The listing builds one solid part. Answer for the finished solid, in the listing's coordinates (mm). Give positions to 0.01 mm unless a question says otherwise; leave off trailing zeros. Write each loop counter-clockwise with the first axis right and the second up, starting at its lowest first coordinate (ties: lowest second). Pieces come first, ordered by that corner, then holes. Notation, with made-up numbers: (51, -28.75) -> (73, -28.75) arc R20 ccw to (73, -11.75) -> close; hole circle Ø1 at (-31, 23). An arc over 180 degrees is marked (long way). One line per question, with ' | ' between items.
from build123d import *

# Parameters (mm, degrees)
SKETCH_1_R          = 1.75
SKETCH_1_R_2        = 1.5
EXTRUDE_1_DEPTH     = 2
SKETCH_2_W          = 27.7
SKETCH_2_H          = 5
CUT_EXTRUDE_1_DEPTH = 10
SKETCH_3_R          = 1.5
CUT_EXTRUDE_2_DEPTH = 10
SKETCH_4_W          = 70
SKETCH_4_H          = 3
EXTRUDE_2_DEPTH     = 2
FILLET_1_R          = 1


with BuildPart() as part:
    # 草图1 → 凸台-拉伸1 (new body)
    with BuildSketch(Plane.XY):
        with BuildLine():
            Line((-35, -27.810744327), (-35, -46.920144927))
            Line((-35, -46.920144927), (35, -46.920144927))
            Line((35, -46.920144927), (35, -27.810744327))
            ThreePointArc((35, -27.810744327), (16.334866743, -2.254950607), (30.958156738, 25.81006644))
            Line((30.958156738, 25.81006644), (35, 32.810744327))
            Line((35, 32.810744327), (35, 46.920144927))
            Line((35, 46.920144927), (16.8, 46.920144927))
            Line((16.8, 46.920144927), (16.8, 51.920144927))
            Line((16.8, 51.920144927), (-10.9, 51.920144927))
            Line((-10.9, 51.920144927), (-10.9, 46.920144927))
            Line((-10.9, 46.920144927), (-35, 46.920144927))
            Line((-35, 46.920144927), (-35, 32.810744327))
            Line((-35, 32.810744327), (-27, 28.191942173))
            Line((-27, 28.191942173), (-27, 23.009508904))
            ThreePointArc((-27, 23.009508904), (-16.614935725, -4.665079356), (-35, -27.810744327))
        make_face()
        with Locations((-16.1979618, -30.0520382)):
            Circle(SKETCH_1_R, mode=Mode.SUBTRACT)
        with Locations((-3.75, 0)):
            Circle(SKETCH_1_R, mode=Mode.SUBTRACT)
        with Locations((16.1979618, -30.0520382)):
            Circle(SKETCH_1_R, mode=Mode.SUBTRACT)
        with Locations((3.75, 0)):
            Circle(SKETCH_1_R, mode=Mode.SUBTRACT)
        with Locations((-16.1979618, 30.0520382)):
            Circle(SKETCH_1_R, mode=Mode.SUBTRACT)
        with Locations((-3.05, 40)):
            Circle(SKETCH_1_R_2, mode=Mode.SUBTRACT)
        with Locations((16.1979618, 30.0520382)):
            Circle(SKETCH_1_R, mode=Mode.SUBTRACT)
        with Locations((11.95, 40)):
            Circle(SKETCH_1_R_2, mode=Mode.SUBTRACT)
    extrude(amount=EXTRUDE_1_DEPTH)

    # 草图2 → 切除-拉伸1 (cut)
    with BuildSketch(Plane(origin=(0, 0, 0), x_dir=(-1, 0, 0), z_dir=(0, 0, -1))):
        with Locations((-2.95, 49.420144927)):
            Rectangle(SKETCH_2_W, SKETCH_2_H)
    extrude(amount=-CUT_EXTRUDE_1_DEPTH, mode=Mode.SUBTRACT)

    # 草图3 → 切除-拉伸2 (cut)
    with BuildSketch(Plane(origin=(0, 0, 0), x_dir=(-1, 0, 0), z_dir=(0, 0, -1))):
        with Locations((-15, 20)):
            Circle(SKETCH_3_R)
        with Locations((15, 20)):
            Circle(SKETCH_3_R)
        with Locations((15, -20)):
            Circle(SKETCH_3_R)
        with Locations((-15, -20)):
            Circle(SKETCH_3_R)
    extrude(amount=-CUT_EXTRUDE_2_DEPTH, mode=Mode.SUBTRACT)

    # 草图4 → 凸台-拉伸2 (add)
    with BuildSketch(Plane(origin=(0, 0, 0), x_dir=(-1, 0, 0), z_dir=(0, 0, -1))):
        with Locations((0, -48.420144927)):
            Rectangle(SKETCH_4_W, SKETCH_4_H)
    extrude(amount=-EXTRUDE_2_DEPTH)

    # 圆角1
    fillet_1_edges = [part.edges().sort_by_distance(p)[0] for p in [
        (35, -49.920144927, 1),
        (-35, -49.920144927, 1),
        (35, -27.810744327, 1),
        (-35, -27.810744327, 1),
        (-27, 23.009508904, 1),
        (-35, 32.810744327, 1),
        (-35, 46.920144927, 1),
        (35, 46.920144927, 1),
    ]]
    fillet(fillet_1_edges, radius=FILLET_1_R)


solid = part.part
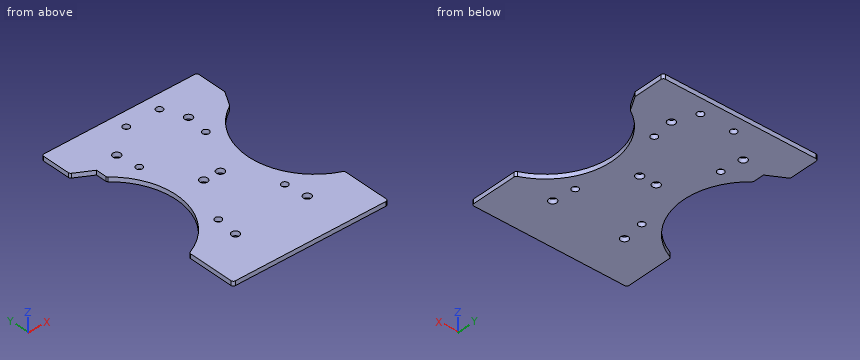
Item 1: Find section A-A (x = 3.75). Write down the section's boundary in (y, z), then the cut area to 3 significant figures.
Answers below:
outline: (-49.92, 0) -> (-1.75, 0) -> (-1.75, 2) -> (-49.92, 2) -> close; (1.75, 0) -> (46.92, 0) -> (46.92, 2) -> (1.75, 2) -> close | area: 187 mm²
Item 2: Find section B-B (y = 40). Write down the section's boundary in (x, z), then the cut area to 3 significant figures.
Answers below:
outline: (-35, 0) -> (-4.55, 0) -> (-4.55, 2) -> (-35, 2) -> close; (-1.55, 0) -> (10.45, 0) -> (10.45, 2) -> (-1.55, 2) -> close; (13.45, 0) -> (35, 0) -> (35, 2) -> (13.45, 2) -> close | area: 128 mm²
Item 3: Find section D-D (x = 11.95). Write down the section's boundary in (y, z).
Answers below:
outline: (-49.92, 0) -> (38.5, 0) -> (38.5, 2) -> (-49.92, 2) -> close; (41.5, 0) -> (46.92, 0) -> (46.92, 2) -> (41.5, 2) -> close
Item 4: Find section C-C (z = 1.2). Count the separate pieces of the cut face and the enclosed holes in it, then the cut area to 3 significant figures.
Answers below:
separate pieces: 1 | enclosed holes: 12 | area: 5,120 mm²
Item 5: Flat-ended cylindrical pins translate along their axes: pin 1 (4.5 mm diameter, centred on x = -16.2, y = -30.05, fed in from +Z); pin 2 (0.6 mm diameter, centred on y = 27, z = 1, fed in from -X). Find the tip coordinate at first contact, or state that the pin passes through.
Answers below:
pin 1: z = 2 | pin 2: x = -27
Item 6: Consider line 1 (Y direction, x = 15, z = 1.1); line 2 (Y direction, x = -3.75, z = 0.95); line 3 (Y direction, x = 15.5, z = 1.2). Determine where each line is inside the solid, lowest interval first. Write a range as [from, to].
Answers below:
line 1: [-49.92, -31.33], [-28.78, -21.5], [-18.5, 18.5], [21.5, 28.78], [31.33, 46.92] | line 2: [-49.92, -1.75], [1.75, 38.67], [41.33, 46.92] | line 3: [-49.92, -31.66], [-28.45, -21.41], [-18.59, 18.59], [21.41, 28.45], [31.66, 46.92]
